Job drawing, mm, ordinate dimensions from the low corner. One solid piece. Give positions to 0.01 mm unless a question says otherwise; leave off trailing zeros. Loops run counter-clockwise (first coordinate to the right, second up) from the corner with the lowest first, then second, coordinate; pieces in that order, holes last. Notation, with made-up numbers: M 2.5,40 L 51.5,40 A16 ccw 51.5,69 Z; hole C 26.25,54 d1. An arc over 180 degrees is marked long. Answer in a Markdown table with one row per item.
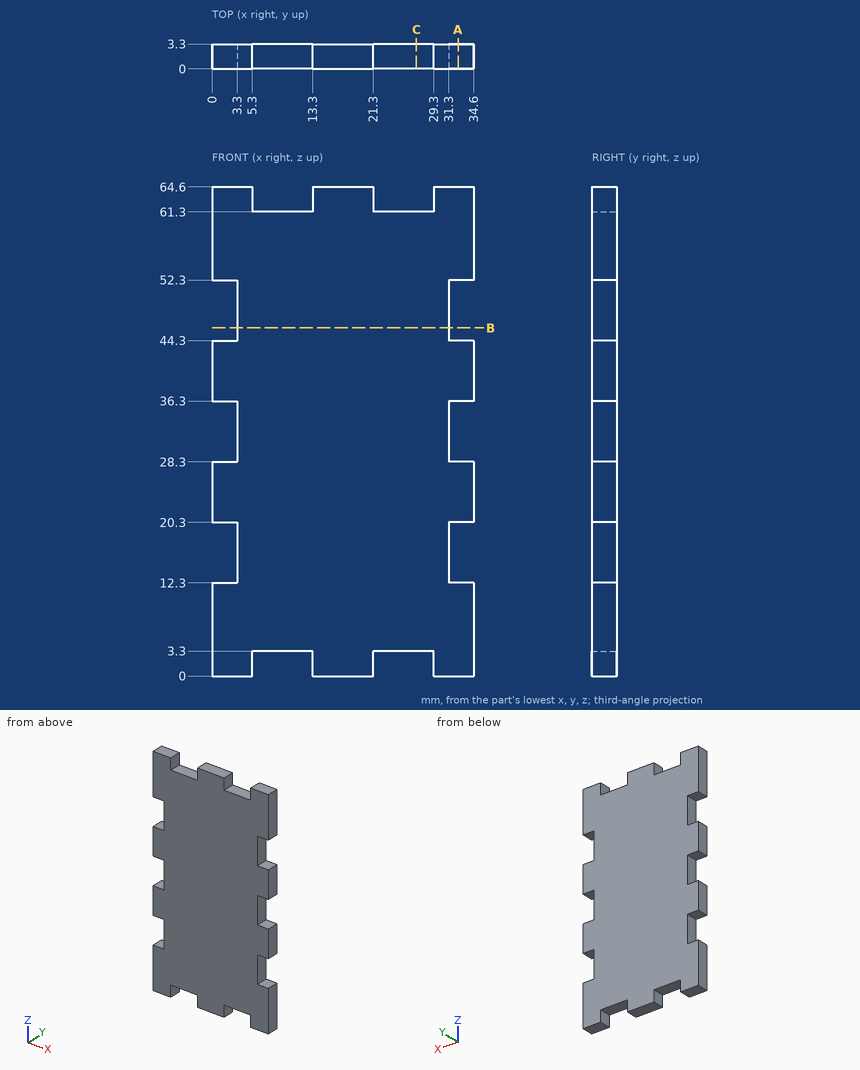
(1) Saw through at C-C (x = 27). Write the cut outline in (y, z).
Recorded:
| item | result |
|---|---|
| outline | M 0,3.3 L 3.3,3.3 L 3.3,61.3 L 0,61.3 Z |
(2) Drill centre lines: line 1 along X through (y, z) = (0.7, 61.5); line 2 along X through (y, z) = (0.4, 34); line 3 along Z through (x, y) = (10, 0.6). Where is each one in solid material? Low to high.
Recorded:
| item | result |
|---|---|
| line 1 | x = 0 to 5.3, 13.3 to 21.3, 29.3 to 34.6 |
| line 2 | x = 3.3 to 31.3 |
| line 3 | z = 3.3 to 61.3 |
(3) Pin check, flat tips, straight feed: pin 1 Ø1.6 at (y, z) = (2, 50) entering from +X; pin 2 Ø1.6 at (x, y) = (8, 1.5) entering from -Z. Stop position of each tip, or through.
Recorded:
| item | result |
|---|---|
| pin 1 | stops at x = 31.3 |
| pin 2 | stops at z = 3.3 |
(4) Saw through at B-B (z = 46). Write the cut outline in (x, y), plus the area to 3 significant figures.
Recorded:
| item | result |
|---|---|
| outline | M 3.3,0 L 31.3,0 L 31.3,3.3 L 3.3,3.3 Z |
| area | 92.4 mm^2 |
(5) Saw through at A-A (x = 32.5). Write the cut outline in (y, z).
Recorded:
| item | result |
|---|---|
| outline | M 0,0 L 3.3,0 L 3.3,12.3 L 0,12.3 Z; M 0,20.3 L 3.3,20.3 L 3.3,28.3 L 0,28.3 Z; M 0,36.3 L 3.3,36.3 L 3.3,44.3 L 0,44.3 Z; M 0,52.3 L 3.3,52.3 L 3.3,64.6 L 0,64.6 Z |
